```python
from build123d import *

# Parameters (mm, degrees)
F0_R     = 3.05
F0_R_2   = 27
F1_DEPTH = 25
F3_DEPTH = 27
F4_R     = 24.536421
F5_DEPTH = 27


with BuildPart() as f1:
    # F0 (on Front) → F1 (new body)
    with BuildSketch(Plane.XZ):
        with BuildLine():
            ThreePointArc((11.511698, 39.871429), (-33.166138, -24.945085), (41.5, 0))
            ThreePointArc((41.5, 0), (33.166138, 24.945085), (11.511698, 39.871429))
        make_face()
        with Locations((-30.310889, -17.5)):
            Circle(F0_R, mode=Mode.SUBTRACT)
        with Locations((0, -35)):
            Circle(F0_R, mode=Mode.SUBTRACT)
        with BuildLine():
            ThreePointArc((32.952267, -19.025), (27.364815, -16.710602), (33.360889, -17.5))
            ThreePointArc((33.360889, -17.5), (33.256963, -18.289398), (32.952267, -19.025))
        make_face(mode=Mode.SUBTRACT)
        with Locations((-30.310889, 17.5)):
            Circle(F0_R, mode=Mode.SUBTRACT)
        Circle(F0_R_2, mode=Mode.SUBTRACT)
        with BuildLine():
            ThreePointArc((32.952267, 19.025), (33.256963, 18.289398), (33.360889, 17.5))
            ThreePointArc((33.360889, 17.5), (27.364815, 16.710602), (32.952267, 19.025))
        make_face(mode=Mode.SUBTRACT)
        with Locations((0, 35)):
            Circle(F0_R, mode=Mode.SUBTRACT)
    extrude(amount=F1_DEPTH)

    # F0 (on Front) → F3 (join)
    with BuildSketch(Plane.XZ):
        Circle(F0_R_2)
    extrude(amount=F3_DEPTH)

    # F4 (on Front) → F5 (cut)
    with BuildSketch(Plane.XZ):
        Circle(F4_R)
    extrude(amount=F5_DEPTH, mode=Mode.SUBTRACT)


solid = f1.part
```
Read the model definition and answer for the solid it produces. Units are mm, in the model's axes. A direction names the side the tool comes from. Coordinates: 2 decimals unless noted, no trailing zeros. Loops run counter-clockwise (first coordinate to the right, second up) from the corner with the lowest first, then second, coordinate; pieces in that order, holes last. Notation, with made-up numbers: (45.5, -27.75) -> (94.5, -27.75) arc R34 cw to (94.5, 3.25) -> close; hole circle Ø2 at (25, -18.75). An arc over 180 degrees is marked (long way). Return JSON: item names as keys, results as strings.
Item 1: For faces 1 (the flat face through (18, 0, -18)), 2 (the flat face through (27, -25, -9)), determine the directions among +Z, -Z, +X, -X, +Y, -Y from which every point of the face is accessible in a straight line to the end or side of a thin tool.
Answers:
{"face 1": "+Z, -Z, +X, -X, +Y", "face 2": "-Y"}
Item 2: Find section A-A (y = -21.5). Determine the outline of the cut face in (x, z) (3 decimals), plus the area to 3 significant figures.
Answers:
{"outline": "(11.512, 39.871) arc R41.5 ccw (long way) to (41.5, 0) arc R41.5 ccw to start; hole circle Ø6.1 at (-30.311, -17.5); hole circle Ø6.1 at (-30.311, 17.5); hole circle Ø49.073 at (0, 0); hole circle Ø6.1 at (0, -35); hole circle Ø6.1 at (0, 35); hole circle Ø6.1 at (30.311, -17.5); hole circle Ø6.1 at (30.311, 17.5)", "area": "3,340 mm2"}
Item 3: Flat-ended cylindrical pins translate along their axes: P1, Ø8, axis at x = -14, y = -18, coming from the -Z side; P2, Ø2, axis at x = -15.5, y = -18, coming from the +Z side; P3, Ø5.5, axis at x = 0, z = 35, coming from the +Y side; P4, Ø1, axis at y = -9.5, z = -14.5, coming from the +X side. Find the tip coordinate at first contact, or state that the pin passes through.
Answers:
{"P1": "stops at z = -40.28", "P2": "stops at z = 38.88", "P3": "passes through", "P4": "stops at x = 39.07"}
Item 4: For a pull along Z with two mould halves and no side action, classify faces 3 (the cylindrical face through (-5.85, -25.99, -26.36)), 4 (the flat face through (6, -27, -24)), 5 (the cylindrical face through (-27.402, -12.325, -16.584)) as +Z half, -Z half, draft (parallel to the pull), parting line (faces both ways), or undercut.
Answers:
{"face 3": "parting line", "face 4": "draft", "face 5": "undercut"}
Item 5: Find section D-D (z = 35). Determine the outline of the cut face in (x, y).
Answers:
{"outline": "(-22.3, -25) -> (-3.05, -25) -> (-3.05, 0) -> (-22.3, 0) -> close; (3.05, -25) -> (22.3, -25) -> (22.3, 0) -> (3.05, 0) -> close"}
Item 6: Find section C-C (z = -5.5). Determine the outline of the cut face in (x, y).
Answers:
{"outline": "(-41.13, -25) -> (-26.43, -25) -> (-26.43, -27) -> (-23.91, -27) -> (-23.91, 0) -> (-41.13, 0) -> close; (23.91, -27) -> (26.43, -27) -> (26.43, -25) -> (41.13, -25) -> (41.13, 0) -> (23.91, 0) -> close"}
Item 7: Find section B-B (x = -7). Determine the outline of the cut face in (y, z).
Answers:
{"outline": "(-27, -26.08) -> (-25, -26.08) -> (-25, -40.91) -> (0, -40.91) -> (0, -23.52) -> (-27, -23.52) -> close; (-27, 23.52) -> (0, 23.52) -> (0, 40.91) -> (-25, 40.91) -> (-25, 26.08) -> (-27, 26.08) -> close"}
Item 8: Find the intervals of material crossed by probe 1 along Z at (x, y) = (0, -16); probe 2 along Z at (x, y) = (-2, -4.5); probe 3 along X at (y, z) = (-20.5, -16), in increasing order.
Answers:
{"probe 1": "z = -41.5 to -38.05, -31.95 to -24.54, 24.54 to 31.95, 38.05 to 41.5", "probe 2": "z = -41.45 to -37.3, -32.7 to -24.45, 24.45 to 32.7, 37.3 to 41.45", "probe 3": "x = -38.29 to -32.97, -27.66 to -18.6, 18.6 to 27.66, 32.97 to 38.29"}
